For this review, take the finished solid that the model builds, in its own axes (mm). A direction names the side the tool comes from. Coordinates: 2 decimals unless noted, no trailing zeros. Loops run counter-clockwise (first coordinate to the right, second up) from the corner with the lowest first, then second, coordinate; pieces in that order, holes last. Notation, with made-up numbers: M 81.25,-9.5 L 123.25,-9.5 A30 cw 123.25,17.5 Z; hole C 72,76 d11. An arc over 180 degrees is marked long. Use one line per item in the form item = value.
```python
from build123d import *
from build123d import SkipClean  # not in build123d's __all__

# Parameters (mm, degrees)
F1_ANGLE_BACK = 90
F1_ANGLE      = 180
F3_ANGLE_BACK = 90
F3_ANGLE      = 180


with BuildPart() as f1:
    # F0 (on Front) → F1 (revolve)
    with BuildSketch(Plane.XZ, mode=Mode.PRIVATE) as f1_sk:
        Polygon((5.425, 0), (0, 0), (0, -72), (6.425, -72), (6.425, -50), (5.425, -50), align=None)
    revolve(f1_sk.sketch.rotate(Axis((0, 0, -36), (0, 0, 1)), -F1_ANGLE_BACK), axis=Axis((0, 0, -36), (0, 0, 1)), revolution_arc=F1_ANGLE)

    # F2 (on Front) → F3 (revolve)
    with BuildSketch(Plane.XZ, mode=Mode.PRIVATE) as f3_sk:
        Polygon((0, -72), (0, 0), (-5.425, 0), (-5.425, -50), (-6.925, -50), (-6.925, -72), align=None)
    revolve(f3_sk.sketch.rotate(Axis((0, 0, -36), (0, 0, 1)), -F3_ANGLE_BACK), axis=Axis((0, 0, -36), (0, 0, 1)), revolution_arc=F3_ANGLE)


solid = f1.part
```
1. Consider section A-A on y = 0. Write out the cut boundary in (x, z) (3 decimals).
Computed values:
outline = M -6.925,-72 L 6.425,-72 L 6.425,-50 L 5.425,-50 L 5.425,0 L -5.425,0 L -5.425,-50 L -6.925,-50 Z
2. Consider section B-B on x = 4.75. Write out the cut boundary in (y, z), plus the area to 3 significant figures.
Computed values:
outline = M -4.33,-72 L 4.33,-72 L 4.33,-50 L 2.62,-50 L 2.62,0 L -2.62,0 L -2.62,-50 L -4.33,-50 Z
area = 452 mm2
3. Consider section D-D on z = -62.5. Write out the cut boundary in (x, y) (3 decimals).
Computed values:
outline = M 0,-6.925 L 0,-6.425 A6.425 ccw 0,6.425 L 0,6.925 A6.925 ccw Z
4. Tool access review of faces 1 (the face through (0, 0, -72)), 2 (the face through (-6, 1, -50)): name each direction out of +Z, -Z, +X, -X, +Y, -Y from which nothing blocks a thin tool from reaching the whole face with its end or side.
Computed values:
face_1 = -Z, +X, -X, +Y, -Y
face_2 = +Z
5. Wall thickness on line 1 along X through (y, z) = (-0.25, -34); line 2 along Z through (x, y) = (-2.5, 5.5): over which ranges is each line inside the solid? List them lowest first. Write a range as from..to.
Computed values:
line_1 = -5.42..5.42
line_2 = -72..-50
6. For pin 1 Ø1.5 at (y, z) = (2, -61) entering from -X; pin 2 Ø8 at (x, z) = (-0.5, -39) entering from +Y (3 decimals), all flat-tipped, find the tip position at first contact; note any pin that passes through.
Computed values:
pin_1 = -6.81
pin_2 = 5.425
7. Consider section C-C on z = -16. Write out the cut boundary in (x, y) (3 decimals), plus the area to 3 significant figures.
Computed values:
outline = C 0,0 d10.85
area = 92.5 mm2
